```python
from build123d import *

# Parameters (mm, degrees)
SKETCH_1_R      = 0.5
EXTRUDE_1_DEPTH = 2


with BuildPart() as part:
    # 草图1 → 凸台-拉伸1 (new body)
    with BuildSketch(Plane.XY):
        with BuildLine():
            Line((12.204680674, 10.819505304), (12.204680674, 5.259215029))
            Line((12.204680674, 5.259215029), (19.479224798, 56.952222064))
            Line((19.479224798, 56.952222064), (35.204680674, 56.952222064))
            ThreePointArc((35.204680674, 56.952222064), (37.192550066, 58.73227825), (35.64190025, 60.903846783))
            Line((35.64190025, 60.903846783), (20.512305514, 64.293307336))
            Line((20.512305514, 64.293307336), (15.841876729, 73.869105416))
            Line((15.841876729, 73.869105416), (17.639464822, 74.74584771))
            Line((17.639464822, 74.74584771), (15.009237941, 80.138611987))
            Line((15.009237941, 80.138611987), (13.211649848, 79.261869694))
            Line((13.211649848, 79.261869694), (9.704680674, 86.452222064))
            Line((9.704680674, 86.452222064), (9.704680674, 82.452222064))
            Line((9.704680674, 82.452222064), (8.204680674, 82.452222064))
            Line((8.204680674, 82.452222064), (8.204680674, 2.569505304))
            Line((8.204680674, 2.569505304), (10.204680674, 2.569505304))
            Line((10.204680674, 2.569505304), (10.204680674, 10.819505304))
            Line((10.204680674, 10.819505304), (12.204680674, 10.819505304))
        make_face()
        with Locations((35.204680674, 58.952222064)):
            Circle(SKETCH_1_R, mode=Mode.SUBTRACT)
    extrude(amount=EXTRUDE_1_DEPTH)


solid = part.part
```
Verification items for the finished model (mm, model axes). A direction names the side the tool comes from. Give positions to 0.01 mm unless a question says otherwise; leave off trailing zeros. Order: outer loops, then holes, each group sorted by start corner. A loop starts at its lowest first (then second) coordinate and runs counter-clockwise, first axis right, second up. Notation, with made-up numbers: (22, 58.5) - (57, 58.5) arc R24 ccw to (57, 80.5) - close; hole circle Ø4 at (46, 12.25). An arc over 180 degrees is marked (long way). Answer as CSV lines item,"result". Start each with the question number.
Item 1: Section check B-B, the plane x = 25.75. Record the boundary of the cut face in (y, z).
Item 2: Material ranges on L1, parallel to X at y = 7.5, z = 0.9; L2, parallel to Y at x = 33.25, z = 0.8; L3, parallel to Y at x = 35, z = 0.6, recorded low to high.
Item 3: Access from +Z, -Z, +X, -X, +Y, -Y to the whole of each face (thin tool, end or side, straight path). Record for faces 1 (the face through (18.21, 69.01, 0.99)), 2 (the face through (10.205, 7, 1)), 3 (the face through (14.123, 79.706, 0.986)), 4 (the face through (9.705, 84, 1)), 5 (the face through (27, 56.952, 1)).
Item 4: Gauge pin test, flat end, axial feed: pin 1 (0.6 mm diameter, centred on y = 85, z = 0.5, fed in from -X). Record the tip position at first contact, or that the pin passes through.
Item 5: Section check C-C, the plane y = 43. Record the boundary of the cut face in (x, z).
Item 6: Mould release check, pull along X, two halves, no side actions. Record for faces 6 (the face through (28.183, 62.575, 0.986)), 7 (the face through (12.205, 8, 1)), 8 (the face through (9, 82.452, 1)): released by +X, released by -X, zero draft, split by the parting line, or undercut.
Item 7: Section check A-A, the plane z = 1.2. Record the boundary of the cut face in (x, y).
Filled in:
1,outline,"(56.95, 0) - (63.12, 0) - (63.12, 2) - (56.95, 2) - close"
2,L1,"8.2 to 10.2, 12.2 to 12.52"
2,L2,"56.95 to 61.44"
2,L3,"56.95 to 58.5, 59.41 to 61.05"
3,face 1,"+Z, -Z, +X"
3,face 2,"+Z, -Z, -Y"
3,face 3,"+Z, -Z, +Y"
3,face 4,"+Z, -Z, -X, +Y"
3,face 5,"+Z, -Z, +X, -Y"
4,pin 1,"x = 9.7"
5,outline,"(8.2, 0) - (17.52, 0) - (17.52, 2) - (8.2, 2) - close"
6,face 6,"released by +X"
6,face 7,"undercut"
6,face 8,"zero draft"
7,outline,"(8.2, 2.57) - (10.2, 2.57) - (10.2, 10.82) - (12.2, 10.82) - (12.2, 5.26) - (19.48, 56.95) - (35.2, 56.95) arc R2 ccw to (35.64, 60.9) - (20.51, 64.29) - (15.84, 73.87) - (17.64, 74.75) - (15.01, 80.14) - (13.21, 79.26) - (9.7, 86.45) - (9.7, 82.45) - (8.2, 82.45) - close; hole circle Ø1 at (35.2, 58.95)"
